Can you work these out from the model? Positions are in its coordinate system, mm. Face numbers are marked on the shaded views. A direction names the side the tool comes from. Round coordinates to 2 decimals unless told otherwise and drop trailing zeros. Order: outer loops, then holes, each group sorted by start corner. A loop starts at its lowest first (then second) coordinate and runs counter-clockwise, first axis right, second up. Notation, with made-up numbers: M 10,67 L 20,67 A15 ccw 20,91 Z; hole C -18,-13 d4. An arc over 180 degrees is marked long. Answer as a JSON object with one key per item and string values. Group by question number.
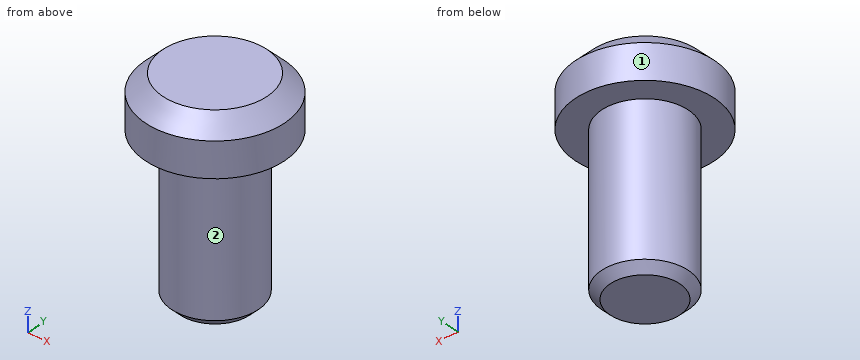
from build123d import *

# Parameters (mm, degrees)
F0_R     = 40
F1_DEPTH = 10
F3_SIZE  = 9.99999
F2_R     = 40
F4_DEPTH = 20
F5_R     = 25
F6_DEPTH = 90
F7_SIZE  = 5


# Not quite as in the source:
# - a fillet or chamfer is up to 0.001 mm smaller than in the source, because OpenCascade refuses the exact size


with BuildPart() as f1:
    # F0 (on Top) → F1 (new body)
    with BuildSketch(Plane.XY):
        Circle(F0_R)
    extrude(amount=F1_DEPTH)

    # F3 (size 10 in the source; OpenCascade refuses exactly that, so slightly less here)
    f3_edges = [f1.edges().sort_by_distance(p)[0] for p in [
        (-40, 0, 10),
    ]]
    chamfer(f3_edges, length=F3_SIZE)

    # F2 (on face) → F4 (join)
    with BuildSketch(Plane(origin=(0, 0, 0), x_dir=(1, 0, 0), z_dir=(0, 0, -1))):
        Circle(F2_R)
    extrude(amount=F4_DEPTH)

    # F5 (on face) → F6 (join)
    with BuildSketch(Plane(origin=(0, 0, -20), x_dir=(1, 0, 0), z_dir=(0, 0, -1))):
        Circle(F5_R)
    extrude(amount=F6_DEPTH)

    # F7
    f7_edges = [f1.edges().sort_by_distance(p)[0] for p in [
        (-25, 0, -110),
    ]]
    chamfer(f7_edges, length=F7_SIZE)


solid = f1.part
Item 1: On a 3-axis mill with a long thin cutter (end or side, diameter ignored), from which of +Z, -Z, +X, -X, +Y, -Y can I reach the whole of each face in a straight line? I mean the marked faces 1 and 2. Say none if no direction works.
Item 2: I'm going to push flat-ended pins straight in: pin 1 Ø2 at (y, z) = (-18, -5) entering from +X; pin 2 Ø6 at (y, z) = (-24.5, -92) entering from +X; pin 3 Ø5 at (x, y) = (31, 0) entering from -Z. Where does each tip first touch, or does it pass through?
Item 3: Suppose I cut it at C-C, the plane z = -38. Write out the boundary of the cut face in (x, y).
Item 4: Suppose I cut it at A-A, the plane y = 0. Write out the boundary of the cut face in (x, z), and give its area (4 significant figures).
Item 5: I need wall thicknesses on line 1 (X direction, y = 1, z = -61); line 2 (X direction, y = -15, z = -59); line 3 (Z direction, x = 36.5, y = 5). Which ranges of each line are inside material? Lowest first, please.
Computed:
{
 "1": {"face 1": "+Z, -Z", "face 2": "-Z"},
 "2": {"pin 1": "stops at x = 36.21", "pin 2": "stops at x = 12.76", "pin 3": "stops at z = -20"},
 "3": {"outline": "C 0,0 d50"},
 "4": {"outline": "M -40,-20 L -25,-20 L -25,-105 L -20,-110 L 20,-110 L 25,-105 L 25,-20 L 40,-20 L 40,0 L 30,10 L -30,10 L -40,0 Z", "area": "6,775 mm^2"},
 "5": {"line 1": "x = -24.98 to 24.98", "line 2": "x = -20 to 20", "line 3": "z = -20 to 3.16"}
}
